Could you check a few things on this model? Use its own coordinates, in mm. A direction names the side the tool comes from. Coordinates: 2 decimals unless noted, no trailing zeros. Order: outer loops, then holes, each group sorted by start corner. A loop starts at its lowest first (then second) coordinate and runs counter-clockwise, first axis right, second up. Notation, with made-up numbers: M 65.5,-39.5 L 79.5,-39.5 A23 cw 79.5,-8.5 Z; hole C -21.5,-17 d6. An arc over 180 degrees is marked long. Write item = value, one per line. Start each with the question number.
from build123d import *

# Parameters (mm, degrees)
SKETCH1_W           = 42
SKETCH1_H           = 42
SKETCH1_W_2         = 36
SKETCH1_H_2         = 36
SKETCH1_R           = 1.45
SKETCH1_R_2         = 11.2
BOSS_EXTRUDE1_DEPTH = 3
BOSS_EXTRUDE2_DEPTH = 25
BOSS_EXTRUDE3_START = -25
SKETCH1_4_W         = 36
SKETCH1_4_H         = 36
SKETCH1_4_R         = 1.45
SKETCH1_4_R_2       = 11.2
BOSS_EXTRUDE3_DEPTH = 3
SKETCH3_R           = 2.2
CUT_EXTRUDE1_DEPTH  = 51.862559904
SKETCH3_3_R         = 6
BOSS_EXTRUDE4_DEPTH = 3
SKETCH2_R           = 2.5
CUT_EXTRUDE2_DEPTH  = 39.820097888
CHAMFER1_SIZE       = 4


with BuildPart() as part:
    # Sketch1 → Boss-Extrude1 (new body)
    # profile 1 of 3: a face of its own
    with BuildSketch(Plane(origin=(0, 0, 0), x_dir=(1, 0, 0), z_dir=(0, 1, 0))):
        Rectangle(SKETCH1_W, SKETCH1_H)
        Rectangle(SKETCH1_W_2, SKETCH1_H_2, mode=Mode.SUBTRACT)
    # profile 2 of 3: a face of its own
    with BuildSketch(Plane(origin=(0, 0, 0), x_dir=(1, 0, 0), z_dir=(0, 1, 0))):
        Rectangle(SKETCH1_W_2, SKETCH1_H_2)
        with Locations(Location((-15.5, -15.5, 0), (0, 0, 270))):
            Circle(SKETCH1_R, mode=Mode.SUBTRACT)
        with Locations(Location((15.5, -15.5, 0), (0, 0, 270))):
            Circle(SKETCH1_R, mode=Mode.SUBTRACT)
        with Locations(Location((15.5, 15.5, 0), (0, 0, 270))):
            Circle(SKETCH1_R, mode=Mode.SUBTRACT)
        with Locations(Location((-15.5, 15.5, 0), (0, 0, 270))):
            Circle(SKETCH1_R, mode=Mode.SUBTRACT)
        with Locations(Location((0, 0, 0), (0, 0, 270))):
            Circle(SKETCH1_R_2, mode=Mode.SUBTRACT)
    # profile 3 of 3: a face of its own
    with BuildSketch(Plane(origin=(0, 0, 0), x_dir=(1, 0, 0), z_dir=(0, 1, 0))):
        Polygon((0, 18), (0, 21), (-21, 21), (-21, -21), (0, -21), (0, -18), (-18, -18), (-18, 18), align=None)
    extrude(amount=BOSS_EXTRUDE1_DEPTH)

    # Sketch1<3> → Boss-Extrude2 (add)
    with BuildSketch(Plane(origin=(0, 0, 0), x_dir=(1, 0, 0), z_dir=(0, 1, 0))):
        Polygon((0, 18), (0, 21), (-21, 21), (-21, -21), (0, -21), (0, -18), (-18, -18), (-18, 18), align=None)
    extrude(amount=-BOSS_EXTRUDE2_DEPTH)

    # Sketch1<4> → Boss-Extrude3 (add)
    # profile 1 of 8: a face of its own
    with BuildSketch(Plane(origin=(0, 0, 0), x_dir=(1, 0, 0), z_dir=(0, 1, 0)).offset(BOSS_EXTRUDE3_START)):
        Polygon((0, 18), (0, 21), (-21, 21), (-21, -21), (0, -21), (0, -18), (-18, -18), (-18, 18), align=None)
    # profile 2 of 8: a face of its own
    with BuildSketch(Plane(origin=(0, 0, 0), x_dir=(1, 0, 0), z_dir=(0, 1, 0)).offset(BOSS_EXTRUDE3_START)):
        Polygon((21, 21), (0, 21), (0, 18), (18, 18), (18, -18), (0, -18), (0, -21), (21, -21), align=None)
    # profile 3 of 8: a face of its own
    with BuildSketch(Plane(origin=(0, 0, 0), x_dir=(1, 0, 0), z_dir=(0, 1, 0)).offset(BOSS_EXTRUDE3_START)):
        Rectangle(SKETCH1_4_W, SKETCH1_4_H)
        with Locations(Location((-15.5, -15.5, 0), (0, 0, 270))):
            Circle(SKETCH1_4_R, mode=Mode.SUBTRACT)
        with Locations(Location((15.5, -15.5, 0), (0, 0, 270))):
            Circle(SKETCH1_4_R, mode=Mode.SUBTRACT)
        with Locations(Location((15.5, 15.5, 0), (0, 0, 270))):
            Circle(SKETCH1_4_R, mode=Mode.SUBTRACT)
        with Locations(Location((-15.5, 15.5, 0), (0, 0, 270))):
            Circle(SKETCH1_4_R, mode=Mode.SUBTRACT)
        with Locations(Location((0, 0, 0), (0, 0, 270))):
            Circle(SKETCH1_4_R_2, mode=Mode.SUBTRACT)
    # profile 4 of 8: a face of its own
    with BuildSketch(Plane(origin=(0, 0, 0), x_dir=(1, 0, 0), z_dir=(0, 1, 0)).offset(BOSS_EXTRUDE3_START)):
        with Locations(Location((-15.5, -15.5, 0), (0, 0, 270))):
            Circle(SKETCH1_4_R)
    # profile 5 of 8: a face of its own
    with BuildSketch(Plane(origin=(0, 0, 0), x_dir=(1, 0, 0), z_dir=(0, 1, 0)).offset(BOSS_EXTRUDE3_START)):
        with Locations(Location((15.5, -15.5, 0), (0, 0, 270))):
            Circle(SKETCH1_4_R)
    # profile 6 of 8: a face of its own
    with BuildSketch(Plane(origin=(0, 0, 0), x_dir=(1, 0, 0), z_dir=(0, 1, 0)).offset(BOSS_EXTRUDE3_START)):
        with Locations(Location((0, 0, 0), (0, 0, 270))):
            Circle(SKETCH1_4_R_2)
    # profile 7 of 8: a face of its own
    with BuildSketch(Plane(origin=(0, 0, 0), x_dir=(1, 0, 0), z_dir=(0, 1, 0)).offset(BOSS_EXTRUDE3_START)):
        with Locations(Location((-15.5, 15.5, 0), (0, 0, 270))):
            Circle(SKETCH1_4_R)
    # profile 8 of 8: a face of its own
    with BuildSketch(Plane(origin=(0, 0, 0), x_dir=(1, 0, 0), z_dir=(0, 1, 0)).offset(BOSS_EXTRUDE3_START)):
        with Locations(Location((15.5, 15.5, 0), (0, 0, 270))):
            Circle(SKETCH1_4_R)
    extrude(amount=BOSS_EXTRUDE3_DEPTH)

    # Sketch3 → Cut-Extrude1 (cut, through all)
    with BuildSketch(Plane(origin=(-18, 0, 0), x_dir=(0, 0, -1), z_dir=(1, 0, 0))):
        with Locations((0, -11)):
            Circle(SKETCH3_R)
    extrude(amount=-CUT_EXTRUDE1_DEPTH, mode=Mode.SUBTRACT)

    # Sketch3<3> → Boss-Extrude4 (add)
    with BuildSketch(Plane(origin=(-18, 0, 0), x_dir=(0, 0, -1), z_dir=(1, 0, 0))):
        with Locations((0, -11)):
            Circle(SKETCH3_3_R)
        Polygon((3.7, -8.863804004), (0, -6.727608008), (-3.7, -8.863804004), (-3.7, -13.136195996), (0, -15.272391992), (3.7, -13.136195996), align=None, mode=Mode.SUBTRACT)
    extrude(amount=BOSS_EXTRUDE4_DEPTH)

    # Sketch2 → Cut-Extrude2 (cut, through all)
    with BuildSketch(Plane(origin=(0, -22, 0), x_dir=(1, 0, 0), z_dir=(0, 1, 0))):
        with Locations(Location((15.5, 15.5, 0), (0, 0, 270))):
            Circle(SKETCH2_R)
        with Locations(Location((15.5, -15.5, 0), (0, 0, 270))):
            Circle(SKETCH2_R)
        with Locations(Location((-15.5, -15.5, 0), (0, 0, 270))):
            Circle(SKETCH2_R)
        with Locations(Location((-15.5, 15.5, 0), (0, 0, 270))):
            Circle(SKETCH2_R)
    extrude(amount=-CUT_EXTRUDE2_DEPTH, mode=Mode.SUBTRACT)

    # Chamfer1
    chamfer1_edges = [part.edges().sort_by_distance(p)[0] for p in [
        (21, 1.5, -21),
        (21, 1.5, 21),
        (21, -23.5, -21),
        (21, -23.5, 21),
    ]]
    chamfer(chamfer1_edges, length=CHAMFER1_SIZE)


solid = part.part
(1) Please list where these lines run through material, in increasing order: probe 1 along X at (y, z) = (-22.8, -15.5); probe 2 along X at (y, z) = (1.15, -15.5); probe 3 along Y at (x, z) = (8.5, 19). Write a range as from..to.
(2) For faces 1 (the cylindrical face through (14, -23.5, -17.5)), 2 (the flat face through (-15, -11, -4)), 3 (the flat face through (0, -11, -19)), which set-ups out of +Z, -Z, +X, -X, +Y, -Y let a thin tool reach every point of the face, with its end or its side?
(3) Imagine slicing it at C-C on x = 8. List the corners of the cut face in (y, z) for me.
(4) Imagine slicing it at B-B on z = 10. List the corners of the cut face in (x, y) for me, plus the area to 3 significant figures.
(5) Thinking about a two-plate mould opening in X: for faces 4 (the flat face through (-17, -11, 3.7)), 5 (the flat face through (19, 1, -19)), 6 (the cylindrical face through (-15.06, 1.48, -14.12)), which applies, released by +X, released by -X, zero draft, split by the parting line, or undercut?
(6) Will these pins go through, and if not, where does the flat tip stop? P1, Ø20, axis at x = 0, z = 0, coming from the +Y side; P2, Ø5.5, axis at y = -11, z = 0, coming from the +X side; P3, Ø1.5, axis at y = -8, z = 5.5, coming from the +X side.
(7) Imagine slicing it at A-A on y = -11. List the corners of the cut face in (x, z) for me, plus the area to 3 significant figures.
(8) Imagine slicing it at D-D on y = -1.25. List the corners of the cut face in (x, z) for me, plus the area to 3 significant figures.
Response:
q1.probe_1 = -21..-18, -13..13, 18..21
q1.probe_2 = -21..-16.95, -14.05..14.05, 16.95..21
q1.probe_3 = -25..-22, 0..3
q2.face_1 = -Y
q2.face_2 = +X
q2.face_3 = +Z, -Z, +X
q3.outline = M -25,-21 L -22,-21 L -22,21 L -25,21 Z; M 0,-21 L 3,-21 L 3,-7.84 L 0,-7.84 Z; M 0,7.84 L 3,7.84 L 3,21 L 0,21 Z
q4.outline = M -21,-25 L 21,-25 L 21,-22 L -18,-22 L -18,0 L -5.04,0 L -5.04,3 L -21,3 Z; M 5.04,0 L 21,0 L 21,3 L 5.04,3 Z
q4.area = 288 mm2
q5.face_4 = zero draft
q5.face_5 = released by +X
q5.face_6 = undercut
q6.P1 = -22
q6.P2 = -18
q6.P3 = -15
q7.outline = M -21,-21 L 0,-21 L 0,-18 L -18,-18 L -18,-6 L -15,-6 L -15,-3.7 L -18,-3.7 L -18,-2.2 L -21,-2.2 Z; M -21,2.2 L -18,2.2 L -18,3.7 L -15,3.7 L -15,6 L -18,6 L -18,18 L 0,18 L 0,21 L -21,21 Z
q7.area = 235 mm2
q8.outline = M -21,-21 L 0,-21 L 0,-18 L -18,-18 L -18,18 L 0,18 L 0,21 L -21,21 Z
q8.area = 234 mm2
